Could you check a few things on this model? Use its own coordinates, in mm. Coordinates: 2 decimals unless noted, no trailing zeros. Loops run counter-clockwise (first coordinate to the right, second up) from the corner with the lowest first, then second, coordinate; pieces in that order, holes last.
from build123d import *

# Parameters (mm, degrees)
F1_DEPTH = 3


# Not quite as in the source:
# - ends of sketch curves that miss each other by under 0.0002 mm in the source are joined


with BuildPart() as f1:
    # F0 (on Front) → F1 (new body)
    with BuildSketch(Plane.XZ):
        with BuildLine():
            Line((17.292411, 22.4886673102), (0, 22.6303943102))
            Line((0, 22.6303943102), (0, -4.0168806898))
            Line((0, -4.0168806898), (7.228795, -4.0700556898))
            Line((7.228795, -4.0700556898), (14.3159177513, -4.5838576898))
            add(Edge.make_bspline(
                [(22.1116757513, -6.0012756898), (19.5885557513, -5.3778676898), (16.9721657513, -4.9410076898), (14.3159177513, -4.5838576898)],
                knots=[0, 0, 0, 0, 1, 1, 1, 1], degree=3))
            add(Edge.make_bspline(
                [(29.0569877513, -8.4108676898), (26.8431947513, -7.4725876898), (24.5259177513, -6.6722926898), (22.1116757513, -6.0012756898)],
                knots=[0, 0, 0, 0, 1, 1, 1, 1], degree=3))
            add(Edge.make_bspline(
                [(34.0179267513, -11.3874226898), (32.6589677513, -10.4530956898), (31.2598277513, -9.5108856898), (29.0569877513, -8.4108676898)],
                knots=[0, 0, 0, 0, 1, 1, 1, 1], degree=3))
            Line((34.0179267513, -11.3874226898), (37.7031947513, -14.7537826898))
            add(Edge.make_bspline(
                [(40.7151917513, -19.7501556898), (39.9025247513, -18.1165876898), (39.0710207513, -16.4798776898), (37.7031947513, -14.7537826898)],
                knots=[0, 0, 0, 0, 1, 1, 1, 1], degree=3))
            add(Edge.make_bspline(
                [(42.3452147513, -26.0221956898), (42.1316587513, -23.8985406898), (41.3798467513, -21.8287056898), (40.7151917513, -19.7501556898)],
                knots=[0, 0, 0, 0, 1, 1, 1, 1], degree=3))
            Line((42.3452147513, -26.0221956898), (63.6418097513, -25.9867956898))
            Line((63.6418097513, -25.9867956898), (63.6418097513, -21.5928156898))
            Line((63.6418097513, -21.5928156898), (85.0611677513, -21.3930906898))
            Line((85.0611677513, -21.3930906898), (85.0783427513, -19.6170306898))
            Line((85.0783427513, -19.6170306898), (94.5155407513, -19.5168076898))
            Line((94.5155407513, -19.5168076898), (99.6440177513, -14.0805456898))
            Line((99.6440177513, -14.0805456898), (98.6518277513, -10.2535206898))
            Line((98.6518277513, -10.2535206898), (95.9587507513, -3.5916906898))
            Line((95.9587507513, -3.5916906898), (91.7065207513, 1.9361993102))
            Line((91.7065207513, 1.9361993102), (86.1786157513, 7.3223693102))
            Line((86.1786157513, 7.3223693102), (79.0915657513, 11.5746073102))
            add(Edge.make_bspline(
                [(66.9018327513, 16.6772693102), (71.1556647513, 15.1125143102), (75.6872037513, 13.6136843102), (79.0915657513, 11.5746073102)],
                knots=[0, 0, 0, 0, 1, 1, 1, 1], degree=3))
            add(Edge.make_bspline(
                [(50.3932967513, 20.4463193102), (56.1680017513, 19.3841543102), (61.5919797513, 18.0714743102), (66.9018327513, 16.6772693102)],
                knots=[0, 0, 0, 0, 1, 1, 1, 1], degree=3))
            add(Edge.make_bspline(
                [(35.1518327513, 22.0634393102), (40.4118917513, 21.7338963102), (45.5332607513, 21.2425493102), (50.3932967513, 20.4463193102)],
                knots=[0, 0, 0, 0, 1, 1, 1, 1], degree=3))
            Line((35.1518327513, 22.0634393102), (17.292411, 22.4886673102))
        make_face()
        with BuildLine():
            add(Edge.make_bspline(
                [(72.7132127513, 5.3379973102), (73.9598487513, 6.5501393102), (75.1615877513, 7.8382423102), (78.0993757513, 6.1884373102)],
                knots=[0, 0, 0, 0, 1, 1, 1, 1], degree=3))
            Line((78.0993757513, 6.1884373102), (84.0525007513, 2.2196843102))
            Line((84.0525007513, 2.2196843102), (89.2969207513, -3.0247356898))
            add(Edge.make_bspline(
                [(89.2969207513, -3.0247356898), (91.9198887513, -8.8158756898), (90.2818957513, -14.5270806898), (82.7768327513, -16.2066456898)],
                knots=[0, 0, 0, 0, 1, 1, 1, 1], degree=3))
            Line((82.7768327513, -16.2066456898), (63.5000457513, -16.2066456898))
            add(Edge.make_bspline(
                [(63.5000457513, -16.2066456898), (57.1380727513, -16.1648706898), (58.7067867513, -12.4673406898), (58.8225907513, -10.9622406898)],
                knots=[0, 0, 0, 0, 1, 1, 1, 1], degree=3))
            Line((58.8225907513, -10.9622406898), (72.7132127513, 5.3379973102))
        make_face(mode=Mode.SUBTRACT)
        with BuildLine():
            add(Edge.make_bspline(
                [(4.2522797513, 13.9133163102), (5.0251887513, 18.5193293102), (9.4633147513, 17.9503943102), (11.1621567513, 15.5787743102)],
                knots=[0, 0, 0, 0, 1, 1, 1, 1], degree=3))
            Line((11.1621567513, 15.5787743102), (20.9422897513, 3.5307823102))
            add(Edge.make_bspline(
                [(20.9422897513, 3.5307823102), (21.3510167513, 2.4878923102), (21.7530967513, 1.2352573102), (19.4311007513, 1.7529523102)],
                knots=[0, 0, 0, 0, 1, 1, 1, 1], degree=3))
            add(Edge.make_bspline(
                [(19.4311007513, 1.7529523102), (15.4182557513, 2.7136493102), (11.2374477513, 2.8345273102), (7.0996287513, 3.1703543102)],
                knots=[0, 0, 0, 0, 1, 1, 1, 1], degree=3))
            add(Edge.make_bspline(
                [(7.0996287513, 3.1703543102), (4.4484227513, 2.8037243102), (4.6391687513, 4.0357343102), (4.2522797513, 5.1962473102)],
                knots=[0, 0, 0, 0, 1, 1, 1, 1], degree=3))
            Line((4.2522797513, 5.1962473102), (4.2522797513, 13.9133163102))
        make_face(mode=Mode.SUBTRACT)
        with BuildLine():
            add(Edge.make_bspline(
                [(20.5525017513, 12.2833043102), (20.0676617513, 14.6816013102), (20.5440417513, 16.3586093102), (24.0960287513, 17.0670743102)],
                knots=[0, 0, 0, 0, 1, 1, 1, 1], degree=3))
            Line((24.0960287513, 17.0670743102), (40.6797337513, 16.2520573102))
            Line((40.6797337513, 16.2520573102), (49.4676807513, 15.1181243102))
            Line((49.4676807513, 15.1181243102), (59.2478147513, 13.4172363102))
            Line((59.2478147513, 13.4172363102), (65.4844207513, 11.8580763102))
            add(Edge.make_bspline(
                [(65.4844207513, 11.8580763102), (67.5337397513, 10.6827963102), (67.6491757513, 8.8628913102), (66.9018317513, 6.7553913102)],
                knots=[0, 0, 0, 0, 1, 1, 1, 1], degree=3))
            Line((66.9018317513, 6.7553913102), (49.8929027513, -14.0805456898))
            add(Edge.make_bspline(
                [(49.8929027513, -14.0805456898), (47.2968437513, -16.6023676898), (45.5455047513, -15.5763756898), (43.9397777513, -13.9388026898)],
                knots=[0, 0, 0, 0, 1, 1, 1, 1], degree=3))
            Line((43.9397777513, -13.9388026898), (20.5525017513, 12.2833043102))
        make_face(mode=Mode.SUBTRACT)
    extrude(amount=F1_DEPTH)

    # F2: F1 across plane


with BuildPart() as f1_1:
    add(f1.part)
    add(f1.part.mirror(Plane.YZ))


solid = f1_1.part
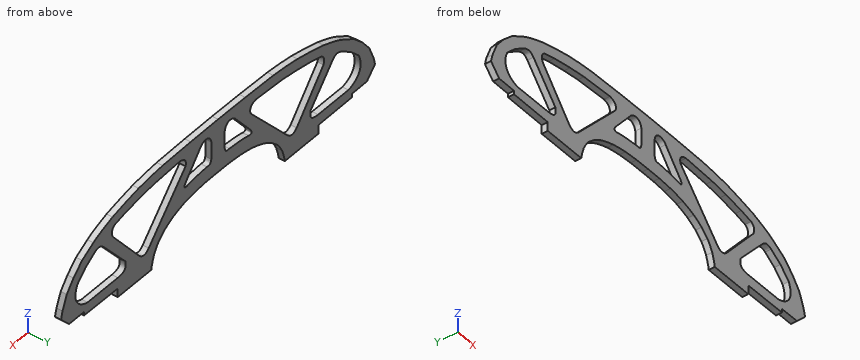
(1) I need wall thicknesses on probe 1 along X at (y, z) = (-1, 10.5); probe 2 along X at (y, z) = (-2.9, -12); probe 3 along X at (y, z) = (-2.25, -15). Which ranges of each line are inside material? Lowest first, please.
Answers:
probe 1: x = -80.88 to -66.92, -22.14 to -15.28, -4.25 to 4.25, 15.28 to 22.14, 66.92 to 80.88
probe 2: x = -99.1 to -89.4, -58.67 to -51.59, -42.21 to -34.69, 34.69 to 42.21, 51.59 to 58.67, 89.4 to 99.1
probe 3: x = -98.78 to -86.14, -59.26 to -48.76, -45.17 to -37.9, 37.9 to 45.17, 48.76 to 59.26, 86.14 to 98.78
(2) For pin 1 (1.5 mm diameter, centred on y = -1, z = 8, fed in from +X); pin 2 (1.5 mm diameter, centred on y = -1.5, z = -24, fed in from +X); pin 3 (1.5 mm diameter, centred on x = -73.5, y = -1, fed in from +Z), each with a flat end and sliding along its axis, tell me the tip position at first contact or that it passes through.
Answers:
pin 1: stops at x = 86.25
pin 2: stops at x = 63.64
pin 3: stops at z = 14.52
(3) Imagine slicing it at B-B, the plane y = -1.25. State how many separate pieces and enclosed holes the cut face has, and give its area (3 significant figures).
Answers:
separate pieces: 1
enclosed holes: 6
area: 3,440 mm2
(4) Imagine slicing it at A-A, the plane z = -1. Write out the boundary of the cut face in (x, y), and give its area (3 significant figures).
Answers:
outline: (-93.97, -3) - (-87.27, -3) - (-87.27, 0) - (-93.97, 0) - close; (-67.31, -3) - (-60.57, -3) - (-60.57, 0) - (-67.31, 0) - close; (-32.4, -3) - (32.4, -3) - (32.4, 0) - (-32.4, 0) - close; (60.57, -3) - (67.31, -3) - (67.31, 0) - (60.57, 0) - close; (87.27, -3) - (93.97, -3) - (93.97, 0) - (87.27, 0) - close
area: 275 mm2
